```python
from build123d import *

# Parameters (mm, degrees)
SKETCH2_W           = 35
SKETCH2_H           = 20
BOSS_EXTRUDE1_DEPTH = 105
SKETCH5_R           = 2
BOSS_EXTRUDE2_DEPTH = 10
FILLET1_R           = 3


with BuildPart() as part:
    # Sketch2 → Boss-Extrude1 (new body)
    with BuildSketch(Plane(origin=(0, 0, 0), x_dir=(1, 0, 0), z_dir=(0, 1, 0))):
        with Locations((17.5, 10)):
            Rectangle(SKETCH2_W, SKETCH2_H)
    extrude(amount=BOSS_EXTRUDE1_DEPTH)

    # Sketch5 → Boss-Extrude2 (add)
    with BuildSketch(Plane(origin=(35, 0, 0), x_dir=(0, 0, -1), z_dir=(1, 0, 0))):
        with Locations(Location((7.9, 103, 0), (0, 0, 90))):
            Circle(SKETCH5_R)
        with Locations(Location((12.1, 103, 0), (0, 0, 90))):
            Circle(SKETCH5_R)
    extrude(amount=BOSS_EXTRUDE2_DEPTH)

    # Fillet1
    fillet1_edges = [part.edges().sort_by_distance(p)[0] for p in [
        (17.5, 105, -20),
        (0, 105, -10),
        (0, 52.5, -20),
        (35, 52.5, -20),
        (35, 52.5, 0),
        (0, 52.5, 0),
        (17.5, 105, 0),
    ]]
    fillet(fillet1_edges, radius=FILLET1_R)


solid = part.part
```
Model file for the job. Use its own axes, mm. A direction names the side the tool comes from. Give positions to 0.01 mm unless a question says otherwise; leave off trailing zeros. Loops run counter-clockwise (first coordinate to the right, second up) from the corner with the lowest first, then second, coordinate; pieces in that order, holes last. Notation, with made-up numbers: (-5.75, 13) -> (8.25, 13) arc R25 cw to (8.25, 41) -> close; hole circle Ø1 at (-3.75, 50.5). An arc over 180 degrees is marked (long way). Use CSV: the item, a comma, the result in double quotes. Start each with the question number.
1) Mould opens along Z. For faces 1 (the cylindrical face through (39.93, 104.908, -11.499)), 2 (the flat face through (17, 50, -20)), 3 (the cylindrical face through (0.86, 51.71, -0.9)) say: released by +Z, released by -Z, zero draft, split by the parting line, or undercut.
2) Slice it at A-A on y = 93. Give the cut face in (x, z), plus the area to 3 significant figures.
3) Wall check: line 1 (X direction, y = 12, z = -9); line 2 (X direction, y = 68, z = -18.75); line 3 (Y direction, x = 40.5, z = -8.25). Give the ranges that are in metal, low to high.
4) Flat gauge pins, fed straight in: pin 1 Ø2 at (y, z) = (58, -5.5) entering from +X; pin 2 Ø2 at (x, z) = (27, -9.5) entering from -Y; pin 3 Ø6 at (x, y) = (37, 66.5) entering from -Z. Where does each tip first touch, or does it go through?
5) Tool access for faces 4 (the cylindrical face through (39.93, 104.908, -7.299)), 5 (the cylindrical face through (19.22, 104.1, -0.86)): list every direction of +Z, -Z, +X, -X, +Y, -Y with a clear straight run to the whole face (end or side of a thin tool).
6) Slice it at B-B on x = 36. Give the cut face in (y, z), plus the area to 3 significant figures.
Computed values:
1,face 1,"undercut"
1,face 2,"released by -Z"
1,face 3,"released by +Z"
2,outline,"(0, -17) arc R3 ccw to (3, -20) -> (32, -20) arc R3 ccw to (35, -17) -> (35, -3) arc R3 ccw to (32, 0) -> (3, 0) arc R3 ccw to (0, -3) -> close"
2,area,"692 mm^2"
3,line 1,"x = 0 to 35"
3,line 2,"x = 0.56 to 34.44"
3,line 3,"y = 101.03 to 104.97"
4,pin 1,"stops at x = 35"
4,pin 2,"stops at y = 0"
4,pin 3,"stops at z = -19.24"
5,face 4,"+X"
5,face 5,"+Z, +X, -X, +Y"
6,outline,"circle Ø4 at (103, -12.1); circle Ø4 at (103, -7.9)"
6,area,"25.1 mm^2"
